```python
from build123d import *

# Parameters (mm, degrees)
SKETCH_1_R          = 60.5
SKETCH_1_R_2        = 1.8
EXTRUDE_1_DEPTH     = 2
SKETCH_2_R          = 1.7
CUT_EXTRUDE_1_DEPTH = 2
FILLET_2_R          = 16
FILLET_3_R          = 10
FILLET_4_R          = 8
FILLET_5_R          = 8
CUT_EXTRUDE_4_DEPTH = 10
FILLET_7_R          = 10
FILLET_8_R          = 10


with BuildPart() as part:
    # 草图1 → 凸台-拉伸1 (new body)
    with BuildSketch(Plane.XY):
        Circle(SKETCH_1_R)
        with Locations((38.537319575, 38.537319575)):
            Circle(SKETCH_1_R_2, mode=Mode.SUBTRACT)
        with Locations((38.537319575, -38.537319575)):
            Circle(SKETCH_1_R_2, mode=Mode.SUBTRACT)
        with Locations((-38.537319575, -38.537319575)):
            Circle(SKETCH_1_R_2, mode=Mode.SUBTRACT)
        with Locations((-38.537319575, 38.537319575)):
            Circle(SKETCH_1_R_2, mode=Mode.SUBTRACT)
    extrude(amount=EXTRUDE_1_DEPTH)

    # 草图2 → 切除-拉伸1 (cut)
    with BuildSketch(Plane.XY.offset(2)):
        with BuildLine():
            Line((-4.375, 0), (-22.789997499, 24.553329998))
            ThreePointArc((-22.789997499, 24.553329998), (-33.5, 0), (-22.789997499, -24.553329998))
            Line((-22.789997499, -24.553329998), (-4.375, 0))
        make_face()
        with BuildLine():
            Line((-22.789997499, 24.553329998), (-32.42566455, 37.400886066))
            ThreePointArc((-32.42566455, 37.400886066), (-49.5, 0), (-32.42566455, -37.400886066))
            Line((-32.42566455, -37.400886066), (-22.789997499, -24.553329998))
            ThreePointArc((-22.789997499, -24.553329998), (-33.5, 0), (-22.789997499, 24.553329998))
        make_face()
        with BuildLine():
            Line((17.189997499, 28.753329998), (26.82566455, 41.600886066))
            ThreePointArc((26.82566455, 41.600886066), (0, 49.5), (-26.82566455, 41.600886066))
            Line((-26.82566455, 41.600886066), (-17.189997499, 28.753329998))
            ThreePointArc((-17.189997499, 28.753329998), (0, 33.5), (17.189997499, 28.753329998))
        make_face()
        with BuildLine():
            Line((0, 5.833333333), (17.189997499, 28.753329998))
            ThreePointArc((17.189997499, 28.753329998), (0, 33.5), (-17.189997499, 28.753329998))
            Line((-17.189997499, 28.753329998), (0, 5.833333333))
        make_face()
        with BuildLine():
            ThreePointArc((49.5, 0), (45.02954805, 20.556989138), (32.42566455, 37.400886066))
            Line((32.42566455, 37.400886066), (22.789997499, 24.553329998))
            ThreePointArc((22.789997499, 24.553329998), (30.705984076, 13.393750106), (33.5, 0))
            ThreePointArc((33.5, 0), (30.705984076, -13.393750106), (22.789997499, -24.553329998))
            Line((22.789997499, -24.553329998), (32.42566455, -37.400886066))
            ThreePointArc((32.42566455, -37.400886066), (45.02954805, -20.556989138), (49.5, 0))
        make_face()
        with BuildLine():
            ThreePointArc((33.5, 0), (30.705984076, 13.393750106), (22.789997499, 24.553329998))
            Line((22.789997499, 24.553329998), (4.375, 0))
            Line((4.375, 0), (22.789997499, -24.553329998))
            ThreePointArc((22.789997499, -24.553329998), (30.705984076, -13.393750106), (33.5, 0))
        make_face()
        with BuildLine():
            ThreePointArc((-26.82566455, -41.600886066), (0, -49.5), (26.82566455, -41.600886066))
            Line((26.82566455, -41.600886066), (17.189997499, -28.753329998))
            ThreePointArc((17.189997499, -28.753329998), (0, -33.5), (-17.189997499, -28.753329998))
            Line((-17.189997499, -28.753329998), (-26.82566455, -41.600886066))
        make_face()
        with BuildLine():
            ThreePointArc((-17.189997499, -28.753329998), (0, -33.5), (17.189997499, -28.753329998))
            Line((17.189997499, -28.753329998), (0, -5.833333333))
            Line((0, -5.833333333), (-17.189997499, -28.753329998))
        make_face()
        with Locations((18, 24)):
            Circle(SKETCH_2_R)
        with Locations((-18, 24)):
            Circle(SKETCH_2_R)
        with Locations((-18, -24)):
            Circle(SKETCH_2_R)
        with Locations((18, -24)):
            Circle(SKETCH_2_R)
    extrude(amount=-CUT_EXTRUDE_1_DEPTH, mode=Mode.SUBTRACT)

    # 圆角2
    fillet_2_edges = [part.edges().sort_by_distance(p)[0] for p in [
        (4.375, 0, 1),
        (-4.375, 0, 1),
    ]]
    fillet(fillet_2_edges, radius=FILLET_2_R)

    # 圆角3
    fillet_3_edges = [part.edges().sort_by_distance(p)[0] for p in [
        (0, -5.833333333, 1),
        (0, 5.833333333, 1),
    ]]
    fillet(fillet_3_edges, radius=FILLET_3_R)

    # 圆角4
    fillet_4_edges = [part.edges().sort_by_distance(p)[0] for p in [
        (26.82566455, -41.600886066, 1),
        (-26.82566455, -41.600886066, 1),
        (-26.82566455, 41.600886066, 1),
        (26.82566455, 41.600886066, 1),
    ]]
    fillet(fillet_4_edges, radius=FILLET_4_R)

    # 圆角5
    fillet_5_edges = [part.edges().sort_by_distance(p)[0] for p in [
        (32.42566455, 37.400886066, 1),
        (32.42566455, -37.400886066, 1),
        (-32.42566455, 37.400886066, 1),
        (-32.42566455, -37.400886066, 1),
    ]]
    fillet(fillet_5_edges, radius=FILLET_5_R)

    # 草图3 → 切除-拉伸4 (cut)
    with BuildSketch(Plane.XY.offset(2)):
        with BuildLine():
            ThreePointArc((-21.124882445, 33.99984326), (-22.40824576, 41.02827952), (-17.563414, 46.279331117))
            ThreePointArc((-17.563414, 46.279331117), (-21.933404034, 44.375396195), (-26.100000126, 42.059957126))
            ThreePointArc((-26.100000126, 42.059957126), (-27.216559114, 41.346207927), (-28.313611465, 40.602825096))
            Line((-28.313611465, 40.602825096), (-21.124882445, 33.99984326))
        make_face()
        with BuildLine():
            ThreePointArc((-17.563414, 46.279331117), (-8.928132775, 48.688175619), (0, 49.5))
            Line((0, 49.5), (0, 60.5))
            ThreePointArc((0, 60.5), (-16.58538253, 58.182257487), (-31.899999898, 51.406614424))
            ThreePointArc((-31.899999898, 51.406614424), (-26.326051556, 51.539531689), (-23.5, 46.733285782))
            ThreePointArc((-23.5, 46.733285782), (-24.1937541, 44.059337326), (-26.100000126, 42.059957126))
            ThreePointArc((-26.100000126, 42.059957126), (-21.933404034, 44.375396195), (-17.563414, 46.279331117))
        make_face()
        with BuildLine():
            Line((0, 60.5), (0, 49.5))
            ThreePointArc((0, 49.5), (8.928132775, 48.688175619), (17.563414, 46.279331117))
            ThreePointArc((17.563414, 46.279331117), (21.933403961, 44.375396231), (26.099999987, 42.059957212))
            ThreePointArc((26.099999987, 42.059957212), (24.32667146, 49.633285844), (31.900000111, 51.406614291))
            ThreePointArc((31.900000111, 51.406614291), (16.585382651, 58.182257453), (0, 60.5))
        make_face()
        with BuildLine():
            ThreePointArc((26.099999987, 42.059957212), (21.933403961, 44.375396231), (17.563414, 46.279331117))
            ThreePointArc((17.563414, 46.279331117), (22.40824576, 41.02827952), (21.124882445, 33.99984326))
            Line((21.124882445, 33.99984326), (28.313611465, 40.602825096))
            ThreePointArc((28.313611465, 40.602825096), (27.216559046, 41.346207972), (26.099999987, 42.059957212))
        make_face()
    extrude(amount=-CUT_EXTRUDE_4_DEPTH, mode=Mode.SUBTRACT)

    # 圆角7
    fillet_7_edges = [part.edges().sort_by_distance(p)[0] for p in [
        (21.124882445, 33.99984326, 1),
        (-21.124882445, 33.99984326, 1),
    ]]
    fillet(fillet_7_edges, radius=FILLET_7_R)

    # 圆角8
    fillet_8_edges = [part.edges().sort_by_distance(p)[0] for p in [
        (28.313611465, 40.602825096, 1),
        (-28.313611465, 40.602825096, 1),
    ]]
    fillet(fillet_8_edges, radius=FILLET_8_R)


solid = part.part
```
Verification items for the finished model (mm, model axes). A direction names the side the tool comes from. Coordinates: 2 decimals unless noted, no trailing zeros. Loops run counter-clockwise (first coordinate to the right, second up) from the corner with the lowest first, then second, coordinate; pieces in that order, holes last. Notation, with made-up numbers: (-33.5, 78.25) -> (16.5, 78.25) arc R12 ccw to (16.5, 96.25) -> close; hole circle Ø4 at (-26, 27). An arc over 180 degrees is marked (long way). Answer in a Markdown table with one row per item. Add a question column.
1. Access from +Z, -Z, +X, -X, +Y, -Y to the whole of each face (thin tool, end or side, straight path). Record for faces 4 (the face through (22.436, -40.929, 0.986)), 5 (the face through (-1, -3, 2)).
2. Section check B-B, the plane y = 5. Enter the section's corners in (x, z), then the cut area to 3 significant figures.
3. Draft check along Y on faces 1 (the face through (-1, -3, 0)), 2 (the face through (-0.1, 12.5, 1)), 3 (the face through (8.376, 0.144, 0.986)). Enter one of: +Y half, -Y half, draft (parallel to the pull), parting line (faces both ways), or undercut.
4. Section check C-C, the plane z = 0.9. Give the number of separate pieces and of enclosed holes in the cut face, then the cut area to 3 significant figures.
5. Material ranges on probe 1 along X at (y, z) = (1, 1.45); probe 2 along Y at (x, z) = (20, 0.9); probe 3 along X at (y, z) = (26, 0.1) (3 decimals), recorded low to high. Write a range as [from, to].
6. Depth check by flat-ended pin: P1, Ø3, axis at x = 18, y = 24, coming from the +Z side. Enter the tip coordinate at first touch or a pass-through.
7. Section check A-A, the plane x = 0. Enter the section's corners in (y, z), then the cut area to 3 significant figures.
Derived:
| question | item | result |
|---|---|---|
| 1 | face 4 | +Z, -Z |
| 1 | face 5 | +Z, +X, -X, +Y, -Y |
| 2 | outline | (-60.29, 0) -> (-49.25, 0) -> (-49.25, 2) -> (-60.29, 2) -> close; (-9.18, 0) -> (9.18, 0) -> (9.18, 2) -> (-9.18, 2) -> close; (49.25, 0) -> (60.29, 0) -> (60.29, 2) -> (49.25, 2) -> close |
| 2 | area | 80.9 mm² |
| 3 | face 1 | draft |
| 3 | face 2 | +Y half |
| 3 | face 3 | undercut |
| 4 | separate pieces | 1 |
| 4 | enclosed holes | 11 |
| 4 | area | 4,760 mm² |
| 5 | probe 1 | x = [-60.49, -49.49], [-8.41, 8.41], [49.49, 60.49] |
| 5 | probe 2 | y = [-57.1, -44.81], [-32.5, -20.83], [20.83, 32.5] |
| 5 | probe 3 | x = [-54.628, -42.122], [-23.875, -15.125], [15.125, 23.875], [42.122, 54.628] |
| 6 | P1 | passes through |
| 7 | outline | (-60.5, 0) -> (-49.5, 0) -> (-49.5, 2) -> (-60.5, 2) -> close; (-12.5, 0) -> (12.5, 0) -> (12.5, 2) -> (-12.5, 2) -> close |
| 7 | area | 72.0 mm² |
